Here's how the part is built. I have some questions about the finished solid (model axes, mm). A direction names the side the tool comes from. Round coordinates to 2 decimals unless told otherwise and drop trailing zeros. Write each loop counter-clockwise with the first axis right and the second up, starting at its lowest first coordinate (ties: lowest second). Pieces come first, ordered by that corner, then holes. Notation, with made-up numbers: M 19.25,-10.5 L 41.25,-10.5 A14 ccw 41.25,-6.5 Z; hole C 41.5,7 d10. An arc over 180 degrees is marked long. Use a Markdown table: item, result. Add a question column.
```python
from build123d import *

# Parameters (mm, degrees)
F0_R     = 9.1
F0_W     = 12.7
F0_H     = 11.5
F1_DEPTH = 14
F3_DEPTH = 5
F5_R     = 17
F5_R_2   = 2
F5_R_3   = 4
F6_DEPTH = 1.5
F2_W     = 12.7
F2_H     = 9
F2_H_2   = 2.5
F8_DEPTH = 3.5


with BuildPart() as f1:
    # F0 (on Top) → F1 (new body)
    with BuildSketch(Plane.XY):
        Circle(F0_R)
        Rectangle(F0_W, F0_H, mode=Mode.SUBTRACT)
    extrude(amount=F1_DEPTH)

    # F2 (on face) → F3 (cut)
    with BuildSketch(Plane(origin=(0, 0, 0), x_dir=(1, 0, 0), z_dir=(0, 0, -1))):
        with BuildLine():
            Line((6.35, -6.5182436285), (6.35, -5.75))
            Line((6.35, -5.75), (-6.35, -5.75))
            Line((-6.35, -5.75), (-6.35, -6.5182436285))
            ThreePointArc((-6.35, -6.5182436285), (-5.1681747735, -7.4899912891), (-3.8402473879, -8.25))
            Line((-3.8402473879, -8.25), (3.8402473879, -8.25))
            ThreePointArc((3.8402473879, -8.25), (5.1681747735, -7.4899912891), (6.35, -6.5182436285))
        make_face()
    extrude(amount=-F3_DEPTH, mode=Mode.SUBTRACT)


with BuildPart() as f6:
    # F5 (on offset) → F6 (new body)
    with BuildSketch(Plane.XY.offset(4)):
        Circle(F5_R)
        with Locations((0, -13.75)):
            Circle(F5_R_2, mode=Mode.SUBTRACT)
        with Locations((0, 5)):
            Circle(F5_R_3, mode=Mode.SUBTRACT)
        with Locations((0, 13.75)):
            Circle(F5_R_2, mode=Mode.SUBTRACT)
    extrude(amount=-F6_DEPTH)

    # F2 (on face) → F8 (cut)
    with BuildSketch(Plane(origin=(0, 0, 0), x_dir=(1, 0, 0), z_dir=(0, 0, -1))):
        with Locations((0, 1.25)):
            Rectangle(F2_W, F2_H)
        with Locations((0, -4.5)):
            Rectangle(F2_W, F2_H_2)
        with BuildLine():
            ThreePointArc((-3.8402473879, -8.25), (-5.1681747735, -7.4899912891), (-6.35, -6.5182436285))
            Line((-6.35, -6.5182436285), (-6.35, -8.25))
            Line((-6.35, -8.25), (-3.8402473879, -8.25))
        make_face()
        with BuildLine():
            Line((6.35, -6.5182436285), (6.35, -5.75))
            Line((6.35, -5.75), (-6.35, -5.75))
            Line((-6.35, -5.75), (-6.35, -6.5182436285))
            ThreePointArc((-6.35, -6.5182436285), (-5.1681747735, -7.4899912891), (-3.8402473879, -8.25))
            Line((-3.8402473879, -8.25), (3.8402473879, -8.25))
            ThreePointArc((3.8402473879, -8.25), (5.1681747735, -7.4899912891), (6.35, -6.5182436285))
        make_face()
        with BuildLine():
            Line((6.35, -8.25), (6.35, -6.5182436285))
            ThreePointArc((6.35, -6.5182436285), (5.1681747735, -7.4899912891), (3.8402473879, -8.25))
            Line((3.8402473879, -8.25), (6.35, -8.25))
        make_face()
    extrude(amount=-F8_DEPTH, mode=Mode.SUBTRACT)


solid = f6.part
```
Item 1: On a 3-axis mill with a long thin cutter (end or side, diameter ignored), from which of +Z, -Z, +X, -X, +Y, -Y can I reach the whole of each face in a straight line? I mean faces 4 (the face through (-0.26, -11.767, 3.26)), 5 (the face through (0, -5.75, 3)). Say none if no direction works.
Item 2: For pin 1 Ø4.5 at (x, y) = (0, -13.75) entering from +Z; pin 2 Ø0.8 at (x, z) = (-1.5, 3) entering from +Y; pin 3 Ø2.5 at (x, y) = (0, 13.75) entering from -Z, each with a flat end and sliding along its axis, tell me the tip position at first contact or that it passes through.
Item 3: Imagine slicing it at B-B on z = 2.85. List the corners of the cut face in (x, y) for me, plus the area to 3 significant figures.
Item 4: Imagine slicing it at D-D on y = 0. List the corners of the cut face in (x, z) for me, plus the area to 3 significant figures.
Item 5: Imagine slicing it at A-A on x = 0. List the corners of the cut face in (y, z) for me, plus the area to 4 significant figures.
Item 6: Imagine slicing it at C-C on y = -13.75. List the corners of the cut face in (x, z) for me, plus the area to 3 significant figures.
Item 7: If we mould it in two halves opening along Y, with no side actions, what happens to faces 1 (the face through (9.139, 14.334, 3.26)), 2 (the face through (2.15, 8.373, 3.594)), 3 (the face through (0, 0, 4))? For each: +Y half, -Y half, draft (parallel to the pull), parting line (faces both ways), or undercut.
Item 8: I need wall thicknesses on probe 1 along Y at (x, z) = (0, 3.05); probe 2 along X at (y, z) = (-12, 2.8); probe 3 along X at (y, z) = (4.5, 2.9). Which ranges of each line are inside material? Lowest first, please. Write a range as from..to.
The answers:
| question | item | result |
|---|---|---|
| 1 | face 4 | +Z, -Z |
| 1 | face 5 | -Z |
| 2 | pin 1 | z = 4 |
| 2 | pin 2 | y = 16.96 |
| 2 | pin 3 | through |
| 3 | outline | C 0,0 d34; hole M -6.35,-5.75 L 6.35,-5.75 L 6.35,8.25 L 2.33,8.25 A4 ccw -2.33,8.25 L -6.35,8.25 Z; hole C 0,-13.75 d4; hole C 0,13.75 d4 |
| 3 | area | 703 mm² |
| 4 | outline | M -17,2.5 L -6.35,2.5 L -6.35,3.5 L 6.35,3.5 L 6.35,2.5 L 17,2.5 L 17,4 L -17,4 Z |
| 4 | area | 38.3 mm² |
| 5 | outline | M -17,2.5 L -15.75,2.5 L -15.75,4 L -17,4 Z; M -11.75,2.5 L -5.75,2.5 L -5.75,3.5 L 1,3.5 L 1,4 L -11.75,4 Z; M 9,2.5 L 11.75,2.5 L 11.75,4 L 9,4 Z; M 15.75,2.5 L 17,2.5 L 17,4 L 15.75,4 Z |
| 5 | area | 20.25 mm² |
| 6 | outline | M -10,2.5 L -2,2.5 L -2,4 L -10,4 Z; M 2,2.5 L 10,2.5 L 10,4 L 2,4 Z |
| 6 | area | 24.0 mm² |
| 7 | face 1 | parting line |
| 7 | face 2 | undercut |
| 7 | face 3 | draft |
| 8 | probe 1 | -17..-15.75, -11.75..-5.75, 9..11.75, 15.75..17 |
| 8 | probe 2 | -12.04..-0.97, 0.97..12.04 |
| 8 | probe 3 | -16.39..-6.35, 6.35..16.39 |
